Source: CAD feature listing. Evaluate the final solid. Frame: model axes, mm. A direction names the side the tool comes from. Round coordinates to 2 decimals unless told otherwise and drop trailing zeros. Order: outer loops, then holes, each group sorted by start corner. A loop starts at its lowest first (then second) coordinate and runs counter-clockwise, first axis right, second up. Notation, with made-up numbers: M 17.5,56 L 27.5,56 A17 cw 27.5,89 Z; hole C -16.5,64 d10. An arc over 180 degrees is marked long. Answer as CSV lines item,"result". Start each with the question number.
Item 1: Pull-direction query (Z, two-part tool) for faces 4 (the face through (11, -176.116, 402)), 5 (the face through (-11, -201, 711.2)), 6 (the face through (-11, 17, 0)); classes: +Z half, -Z half, draft (parallel to the pull), parting line (faces both ways), or undercut.
Item 2: First-contact query: P1, Ø5, axis at x = 211.5, z = 571, coming from the +Y side; P2, Ø2, axis at x = 524, z = 564.5, coming from the -Y side; P3, Ø10, axis at x = -586, y = -7.5, coming from the +Z side. Flat tips, straight axial feed; report the tip coordinate or a pass-through.
Item 3: Section query A-A on x = 52. Return the cut outline in (y, z).
Item 4: Set-up query: faces 1 (the face through (11, -1219.2, 50)), 2 (the face through (-11, -226.916, 402)), 3 (the face through (-11, 531, 101.6)). Return all of +Z, -Z, +X, -X, +Y, -Y with unobstructed straight access to the full face (end or side cutting, diameter ignored); none if empty.
Item 5: Line query: line 1 (Z direction, x = 153.5, y = 809.5); line 2 (Y direction, x = -695, z = 312). Output: solid intervals per line, ascending. Write a range as [from, to].
Item 6: Section query B-B on z = 282.5. Return the cut outline in (x, y), plus the area to 3 significant figures.
Item 7: Section query C-C on y = -554. Return the cut outline in (x, z).
Autodesk Inventor part; units mm, degrees
ref_plane "YZ Plane" through (0, 0, 0) normal (1, 0, 0) x (0, 1, 0)
ref_plane "XZ Plane" through (0, 0, 0) normal (0, 1, 0) x (-1, 0, 0)
ref_plane "XY Plane" through (0, 0, 0) normal (0, 0, 1) x (1, 0, 0)
sketch "Sketch1" plane through (0, 0, 0) normal (0, 0, 1) x (1, 0, 0)
  line L0 (762, -1219.2) -> (-762, -1219.2)
  line L1 (-762, -1219.2) -> (-762, 1219.2)
  line L2 (-762, 1219.2) -> (762, 1219.2)
  line L3 (762, 1219.2) -> (762, -1219.2)
  line L4 (762, -1219.2) -> (-762, 1219.2) construction
  line L5 (-762, -1219.2) -> (762, 1219.2) construction
  point P0 (0, 0)
  dimension "d0" = 1524
  dimension "d5" = 2438.4
extrude "Extrusion1" add sketch "Sketch1" along normal blind 101.6
sketch "Sketch2" plane through (0, 0, 101.6) normal (0, 0, 1) x (1, 0, 0)
  line L0 (-762, -226.9161) -> (762, -226.9161)
  line L1 (762, -226.9161) -> (762, -176.1161)
  line L2 (762, -176.1161) -> (-762, -176.1161)
  line L3 (-762, -176.1161) -> (-762, -226.9161)
  line L4 (-762, 1219.2) -> (-762, -1219.2)
  point P0 (0, 0)
  dimension "d6" = 50.8
  dimension "d7" = 1524
  dimension "d8" = 0
extrude "Extrusion2" add sketch "Sketch2" along normal blind 609.6
properties part number "Wall_desk"
Results:
1,face 4,"draft"
1,face 5,"+Z half"
1,face 6,"-Z half"
2,P1,"y = -176.12"
2,P2,"y = -226.92"
2,P3,"z = 101.6"
3,outline,"M -1219.2,0 L 1219.2,0 L 1219.2,101.6 L -176.12,101.6 L -176.12,711.2 L -226.92,711.2 L -226.92,101.6 L -1219.2,101.6 Z"
4,face 1,"+Z, -Z, +X, -X, -Y"
4,face 2,"+Z, +X, -X, -Y"
4,face 3,"+Z, +X, -X, +Y"
5,line 1,"[0, 101.6]"
5,line 2,"[-226.92, -176.12]"
6,outline,"M -762,-226.92 L 762,-226.92 L 762,-176.12 L -762,-176.12 Z"
6,area,"77,400 mm^2"
7,outline,"M -762,0 L 762,0 L 762,101.6 L -762,101.6 Z"
